from build123d import *

# Parameters (mm, degrees)
SKETCH1_W                 = 304.8
SKETCH1_H                 = 152.4
BOSS_EXTRUDE1_DEPTH       = 6.35
M4X0_7_TAPPED_HOLE1_D     = 3.3
M4X0_7_TAPPED_HOLE1_DEPTH = 10.1
M4X0_7_TAPPED_HOLE1_TIP   = 1.65
SKETCH5_R                 = 3.375
CUT_EXTRUDE1_DEPTH        = 7.35
SKETCH6_R                 = 1.65
CUT_EXTRUDE2_DEPTH        = 7.35
SKETCH7_R                 = 1.65
CUT_EXTRUDE3_DEPTH        = 7.35


with BuildPart() as part:
    # Sketch1 → Boss-Extrude1 (new body)
    with BuildSketch(Plane.XY):
        Rectangle(SKETCH1_W, SKETCH1_H)
    extrude(amount=BOSS_EXTRUDE1_DEPTH)

    # M4x0.7 Tapped Hole1
    with Locations(Plane(origin=(78.4, 49.7, 0), x_dir=(-1, 0, 0), z_dir=(0, 0, -1))):
        with Locations((0, 0), (0, -26), (-28, -26), (-28, 0), (0, -73.4), (0, -99.4), (-28, -73.4), (-28, -99.4), (184.8, 0), (156.8, 0), (156.8, -26), (184.8, -26), (184.8, -73.4), (184.8, -99.4), (156.8, -73.4), (156.8, -99.4)):
            Hole(M4X0_7_TAPPED_HOLE1_D / 2, depth=M4X0_7_TAPPED_HOLE1_DEPTH)
            with Locations((0, 0, -(M4X0_7_TAPPED_HOLE1_DEPTH + M4X0_7_TAPPED_HOLE1_TIP / 2))):  # 90° drill point
                Cone(0, M4X0_7_TAPPED_HOLE1_D / 2, M4X0_7_TAPPED_HOLE1_TIP, mode=Mode.SUBTRACT)

    # Sketch5 → Cut-Extrude1 (cut, through all)
    with BuildSketch(Plane.XY.offset(6.35)):
        with Locations((-117.4, -50.000126651)):
            Circle(SKETCH5_R)
        with Locations((-117.4, 49.999873349)):
            Circle(SKETCH5_R)
        with Locations((-17.4, -50.000126651)):
            Circle(SKETCH5_R)
        with Locations((-17.4, 49.999873349)):
            Circle(SKETCH5_R)
    extrude(amount=-CUT_EXTRUDE1_DEPTH, mode=Mode.SUBTRACT)

    # Sketch6 → Cut-Extrude2 (cut, through all)
    with BuildSketch(Plane(origin=(0, 0, 0), x_dir=(-1, 0, 0), z_dir=(0, 0, -1))):
        with Locations((33, -69.2)):
            Circle(SKETCH6_R)
        with Locations((33, -23.2)):
            Circle(SKETCH6_R)
        with Locations((-33, -23.2)):
            Circle(SKETCH6_R)
        with Locations((-33, -69.2)):
            Circle(SKETCH6_R)
    extrude(amount=-CUT_EXTRUDE2_DEPTH, mode=Mode.SUBTRACT)

    # Sketch7 → Cut-Extrude3 (cut, through all)
    with BuildSketch(Plane.XY.offset(6.35)):
        with Locations((122.4, 15)):
            Circle(SKETCH7_R)
        with Locations((122.4, -15)):
            Circle(SKETCH7_R)
    extrude(amount=-CUT_EXTRUDE3_DEPTH, mode=Mode.SUBTRACT)


solid = part.part
Read the model definition and answer for the solid it produces. Units are mm, in the model's axes. Give positions to 0.01 mm unless a question says otherwise; leave off trailing zeros. Loops run counter-clockwise (first coordinate to the right, second up) from the corner with the lowest first, then second, coordinate; pieces in that order, holes last. Notation, with made-up numbers: (-36.75, 25.25) -> (-12.75, 25.25) arc R22 ccw to (-12.75, 33.25) -> close; hole circle Ø9 at (82, 7). An arc over 180 degrees is marked (long way). Answer as CSV lines item,"result".
Item 1: Consider line 1 (Y direction, x = 78.4, z = 3); line 2 (Y direction, x = 122.4, z = 4.5); line 3 (Y direction, x = -18.5, z = 1). Determine where each line is inside the solid, lowest interval first. Write a range as [from, to].
Returned:
line 1,"y = [-76.2, -51.35], [-48.05, -25.35], [-22.05, 22.05], [25.35, 48.05], [51.35, 76.2]"
line 2,"y = [-76.2, -16.65], [-13.35, 13.35], [16.65, 76.2]"
line 3,"y = [-76.2, -53.19], [-46.81, 46.81], [53.19, 76.2]"
Item 2: Find section A-A on x = -17.4. Give the vertices of the cut face in (y, z), plus the area to 3 significant figures.
Returned:
outline,"(-76.2, 0) -> (-53.38, 0) -> (-53.38, 6.35) -> (-76.2, 6.35) -> close; (-46.63, 0) -> (46.62, 0) -> (46.62, 6.35) -> (-46.63, 6.35) -> close; (53.37, 0) -> (76.2, 0) -> (76.2, 6.35) -> (53.37, 6.35) -> close"
area,"882 mm²"
Item 3: Determine the mould class of faces 1 (the face through (-152.4, -1, 3)), 2 (the face through (-114.18, 51.01, 3.22)), 3 (the face through (-2, -76.2, 3)) for opening direction Y: +Y half, -Y half, draft (parallel to the pull), parting line (faces both ways), or undercut.
Returned:
face 1,"draft"
face 2,"undercut"
face 3,"-Y half"
Item 4: This flat-tipped pin is pushed along its axis until it touches: pin 1 (5.5 mm diameter, centred on x = -106.4, y = 23.7, fed in from -Z). Where does it stop, or does it pass through?
Returned:
pin 1,"stops at z = 0"
